from build123d import *

# Parameters (mm, degrees)
F0_W     = 140
F0_H     = 59
F1_DEPTH = 3.3
F2_W     = 111.440674
F2_H     = 1.685995
F3_DEPTH = 25
F4_W     = 27.34
F4_H     = 19
F5_DEPTH = 25
F6_W     = 27.34
F6_H     = 26.557377
F7_DEPTH = 25
F8_R     = 1.5
F9_DEPTH = 3


with BuildPart() as f1:
    # F0 (on Front) → F1 (new body)
    with BuildSketch(Plane.XZ):
        Rectangle(F0_W, F0_H)
        Polygon((85, -29.5), (70, 29.5), (70, -29.5), align=None)
    extrude(amount=F1_DEPTH)

    # F2 (on face) → F3 (cut)
    with BuildSketch(Plane.XZ.offset(3.3)):
        with Locations((0, -9.62422)):
            Rectangle(F2_W, F2_H)
    extrude(amount=-F3_DEPTH, mode=Mode.SUBTRACT)

    # F4 (on face) → F5 (cut)
    with BuildSketch(Plane.XZ.offset(3.3)):
        with Locations((42.050337, 12.718777)):
            Rectangle(F4_W, F4_H)
    extrude(amount=-F5_DEPTH, mode=Mode.SUBTRACT)

    # F6 (on face) → F7 (cut)
    with BuildSketch(Plane.XZ.offset(3.3)):
        with Locations((42.050337, 13.278688)):
            Rectangle(F6_W, F6_H)
    extrude(amount=-F7_DEPTH, mode=Mode.SUBTRACT)

    # F8 (on face) → F9 (cut)
    with BuildSketch(Plane(origin=(0, 0, 0), x_dir=(-1, 0, 0), z_dir=(0, 1, 0))):
        with Locations((55, 14.5)):
            Circle(F8_R)
        with Locations((62, -9.5)):
            Circle(F8_R)
        with Locations((-63, -9.5)):
            Circle(F8_R)
        with Locations((-63, 14.5)):
            Circle(F8_R)
    extrude(amount=-F9_DEPTH, mode=Mode.SUBTRACT)


solid = f1.part
Verification items for the finished model (mm, model axes). A direction names the side the tool comes from. Give positions to 0.01 mm unless a question says otherwise; leave off trailing zeros. Loops run counter-clockwise (first coordinate to the right, second up) from the corner with the lowest first, then second, coordinate; pieces in that order, holes last. Notation, with made-up numbers: (-1.75, 16.5) - (17.25, 16.5) arc R17 ccw to (17.25, 22.5) - close; hole circle Ø5 at (6.25, -34.5). An arc over 180 degrees is marked (long way). Write item = value, one per line. Start each with the question number.
Q1. Cross-section at B-B, the plane y = -1.2. Enter the section's corners in (x, z).
Q2. Cross-section at A-A, the plane x = -36. Enter the section's corners in (y, z).
Q3. Cross-section at D-D, the plane x = 45.5. Enter the section's corners in (y, z), and give its area (3 significant figures).
Q4. Tool access check on faces 1 (the face through (61.614, -1.479, -10.075)), 2 (the face through (-1, -2, -10.467)), 3 (the face through (77.6, -1.6, -0.4)). Record the directions out of +Z, -Z, +X, -X, +Y, -Y that give a thin tool (end or side, any length) a straight path to the whole face; none if there is none.
Q5. Depth check by flat-ended pin: P1, Ø0.9, axis at x = 62.5, z = -9.5, coming from the +Y side; P2, Ø0.8, axis at y = -2, z = -9.5, coming from the +X side. Enter the tip coordinate at first touch or a pass-through.
Q6. Cross-section at C-C, the plane z = 14.5. Enter the section's corners in (x, y).
Q7. Mould release check, pull along Z, two halves, no side actions. Record for faces 4 (the face through (6, -2, -29.5)), 5 (the face through (-1, -2, 29.5)), 6 (the face through (-1, -2, -8.781)): released by +Z, released by -Z, zero draft, split by the parting line, or undercut.
Q8. Thickness scan on line 1 (Z direction, x = 54, y = -2.45); line 2 (Z direction, x = -55, y = -1.25); line 3 (Z direction, x = -62, y = -1). Record the ranges inside material, lowest first.
Answer key:
q1.outline = (-70, -29.5) - (85, -29.5) - (70, 29.5) - (-70, 29.5) - close; hole circle Ø3 at (-62, -9.5); hole circle Ø3 at (-55, 14.5); hole (-55.72, -10.47) - (55.72, -10.47) - (55.72, -8.78) - (-55.72, -8.78) - close; hole (28.38, 0) - (55.72, 0) - (55.72, 26.56) - (28.38, 26.56) - close; hole circle Ø3 at (63, -9.5); hole circle Ø3 at (63, 14.5)
q2.outline = (-3.3, -29.5) - (0, -29.5) - (0, -10.47) - (-3.3, -10.47) - close; (-3.3, -8.78) - (0, -8.78) - (0, 29.5) - (-3.3, 29.5) - close
q3.outline = (-3.3, -29.5) - (0, -29.5) - (0, -10.47) - (-3.3, -10.47) - close; (-3.3, -8.78) - (0, -8.78) - (0, 0) - (-3.3, 0) - close; (-3.3, 26.56) - (0, 26.56) - (0, 29.5) - (-3.3, 29.5) - close
q3.area = 101 mm^2
q4.face_1 = +Y
q4.face_2 = +Y, -Y
q4.face_3 = +Z, +X, +Y, -Y
q5.P1 = -3
q5.P2 = 80.02
q6.outline = (-70, -3.3) - (28.38, -3.3) - (28.38, 0) - (-53.5, 0) - (-53.5, -3) - (-56.5, -3) - (-56.5, 0) - (-70, 0) - close; (55.72, -3.3) - (73.81, -3.3) - (73.81, 0) - (64.5, 0) - (64.5, -3) - (61.5, -3) - (61.5, 0) - (55.72, 0) - close
q7.face_4 = released by -Z
q7.face_5 = released by +Z
q7.face_6 = undercut
q8.line_1 = -29.5 to -10.47, -8.78 to 0, 26.56 to 29.5
q8.line_2 = -29.5 to -10.47, -8.78 to 13, 16 to 29.5
q8.line_3 = -29.5 to -11, -8 to 29.5
